Autodesk Inventor part; units mm, degrees
ref_plane "YZ Plane" through (0, 0, 0) normal (1, 0, 0) x (0, 1, 0)
ref_plane "XZ Plane" through (0, 0, 0) normal (0, 1, 0) x (-1, 0, 0)
ref_plane "XY Plane" through (0, 0, 0) normal (0, 0, 1) x (1, 0, 0)
sketch "Sketch1" plane through (0, 0, 0) normal (0, 0, 1) x (1, 0, 0)
  line L0 (0, 0) -> (3.175, 0)
  line L1 (3.175, 0) -> (3.175, 25.4)
  line L2 (3.175, 25.4) -> (0, 25.4)
  line L3 (0, 25.4) -> (0, 0)
  line L4 (0, 0) -> (25.4, 0)
  line L5 (25.4, 0) -> (25.4, 3.175)
  line L6 (25.4, 3.175) -> (0, 3.175)
  line L7 (0, 3.175) -> (0, 0)
  dimension "d0" = 3.175
  dimension "d1" = 25.4
  dimension "d2" = 25.4
  dimension "d3" = 3.175
extrude "Extrusion1" add sketch "Sketch1" along normal blind 50.8
sketch "Sketch2" plane through (3.175, 3.175, 0) normal (0, 1, 0) x (1, 0, 0)
  line L0 (-3.175, -50.8) -> (22.225, -50.8) construction
  line L1 (-3.175, -50.8) -> (13.462, -50.8) construction
  line L2 (13.462, -50.8) -> (13.462, -31.75) construction
  line L3 (13.462, -50.8) -> (32.512, -50.8) construction
  circle A0 centre (13.462, -31.75) radius 6.35
  point P0 (-3.175, 0)
  dimension "d6" = 16.637
  dimension "d7" = 19.05
  dimension "d8" = 90
  dimension "d9" = 12.7
extrude "Extrusion2" cut sketch "Sketch2" against normal blind 50.8
sketch "Sketch3" plane through (3.175, 3.175, 0) normal (0, 1, 0) x (1, 0, 0)
  circle A0 centre (13.462, -31.75) radius 6.35 construction
  line L0 (13.462, -31.75) -> (13.462, -42.2402) construction
  line L1 (13.462, -42.2402) -> (13.462, -13.7414) construction
  circle A1 centre (13.462, -42.2402) radius 1.7018
  circle A2 centre (13.462, -13.7414) radius 1.7018
  point P0 (-3.175, 0)
  dimension "d12" = 10.4902
  dimension "d13" = 28.4988
  dimension "d14" = 3.4036
  dimension "d15" = 3.4036
extrude "Extrusion3" cut sketch "Sketch3" against normal blind 50.8
sketch "Sketch4" plane through (3.175, 3.175, 0) normal (1, 0, 0) x (0, 0, -1)
  line L0 (0, 0) -> (0, 22.225) construction
  line L1 (0, 22.225) -> (-12.7, 22.225) construction
  line L2 (0, 22.225) -> (-50.8, 22.225) construction
  line L3 (-12.7, 22.225) -> (-12.7, 9.525) construction
  line L4 (-12.7, 9.525) -> (-38.1, 9.525) construction
  circle A0 centre (-12.7, 9.525) radius 2.5797
  circle A1 centre (-38.1, 9.525) radius 2.5797
  point P0 (0, -3.175)
  dimension "d18" = 12.7
  dimension "d19" = 12.7
  dimension "d20" = 25.4
  dimension "d21" = 5.1594
extrude "Extrusion4" cut sketch "Sketch4" against normal blind 50.8
properties part number "2in L-Bracket"
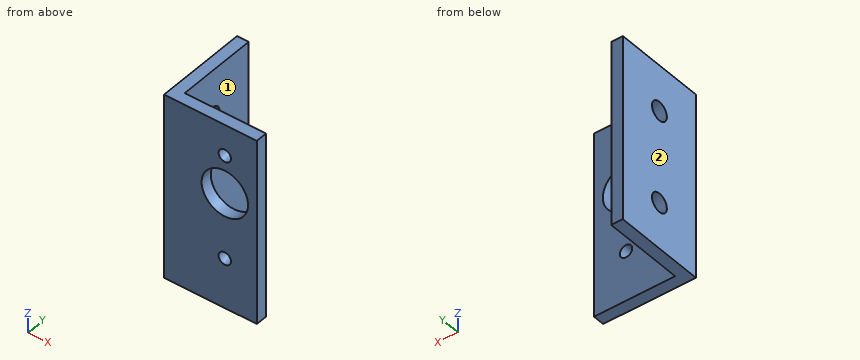
Model file for the job. Use its own axes, mm. Face numbers are marked on the shaded views. A direction names the side the tool comes from. Coordinates: 2 decimals unless noted, no trailing zeros. Write each loop counter-clockwise with the first axis right and the second up, starting at its lowest first coordinate (ties: lowest second). Pieces come first, ordered by that corner, then holes. Notation, with made-up numbers: (-25, -17.5) - (-21, -17.5) arc R34 cw to (-21, 14.5) - close; hole circle Ø2 at (39, 28.5). An arc over 180 degrees is marked (long way). One line per question, with ' | ' between items. Start each with the question number.
Q1. 3-axis set-ups, long thin cutter, end or side, ignore diameter. For the marked faces 1 and 2: which of +Z, -Z, +X, -X, +Y, -Y reach the whole face in a straight line?
Q2. Cut at C-C, the plane y = 12.7. List the corners of the cut face in (x, z) (3 decimals).
Q3. Drill centre lines: line 1 (Y direction, x = 2.15, z = 38.1); line 2 (X direction, y = 1, z = 31.75); line 3 (Y direction, x = 11, z = 25.5) (3 decimals). Where is each one in solid material? Low to high. Write a range as [from, to].
Q4. Cut at D-D, the plane z = 13. List the corners of the cut face in (x, y) (3 decimals).
Q5. Cut at B-B, the plane z = 31.75. List the corners of the cut face in (x, y) (3 decimals), then the cut area to 3 significant figures.
Q6. Cut at A-A, the plane x = 15.5. List the corners of the cut face in (y, z) (3 decimals), then the cut area to 3 significant figures.
Q7. Pin check, flat tips, straight feed: pin 1 (4 mm diameter, centred on y = 12, z = 42.5, fed in from -X); pin 2 (6.5 mm diameter, centred on y = 12.7, z = 38.1, fed in from +X) (3 decimals). Stop position of each tip, or through.
Answer below:
1) face 1: +Z, -Z, +X, +Y | face 2: +Z, -Z, -X, +Y, -Y
2) outline: (0, 0) - (3.175, 0) - (3.175, 10.12) - (0, 10.12) - close; (0, 15.28) - (3.175, 15.28) - (3.175, 35.52) - (0, 35.52) - close; (0, 40.68) - (3.175, 40.68) - (3.175, 50.8) - (0, 50.8) - close
3) line 1: [0, 10.12], [15.28, 25.4] | line 2: [0, 10.29], [22.99, 25.4] | line 3: [0, 3.175]
4) outline: (0, 0) - (15.105, 0) - (15.105, 3.175) - (3.175, 3.175) - (3.175, 10.138) - (0, 10.138) - close; (0, 15.262) - (3.175, 15.262) - (3.175, 25.4) - (0, 25.4) - close; (18.169, 0) - (25.4, 0) - (25.4, 3.175) - (18.169, 3.175) - close
5) outline: (0, 0) - (10.287, 0) - (10.287, 3.175) - (3.175, 3.175) - (3.175, 25.4) - (0, 25.4) - close; (22.987, 0) - (25.4, 0) - (25.4, 3.175) - (22.987, 3.175) - close | area: 111 mm^2
6) outline: (0, 0) - (3.175, 0) - (3.175, 12.475) - (0, 12.475) - close; (0, 15.008) - (3.175, 15.008) - (3.175, 25.503) - (0, 25.503) - close; (0, 37.997) - (3.175, 37.997) - (3.175, 40.974) - (0, 40.974) - close; (0, 43.506) - (3.175, 43.506) - (3.175, 50.8) - (0, 50.8) - close | area: 106 mm^2
7) pin 1: x = 0 | pin 2: x = 3.175
